Study the drawing (mm; zero at the part's minimum x, y, z) and answer. A direction names the side the tool comes from. Give positions to 0.01 mm unless a question says otherwise; leave off trailing zeros. Order: outer loops, then holes, each group sorted by start corner. A loop starts at its lowest first (then second) coordinate and runs counter-clockwise, first axis right, second up. Notation, with made-up numbers: (67.25, 3.25) - (119.25, 3.25) arc R37 ccw to (119.25, 40.25) - close; hole circle Ø7 at (77.25, -23.75). An arc over 180 degrees is marked (long way). Write each question's results on one line, items separated by ' | '. Start each with the question number.
1. Section D-D (z = 1.25) is taken. Give the vertices of the cut face in (x, y), and give its area (3 significant figures).
2. Find the intervals of material crossed by L1, parallel to X at y = 9.75, z = 2.25; L2, parallel to Z at x = 3.75, y = 16.75; L3, parallel to Z at x = 9, y = 9.25, in increasing order.
3. Determine the mould class of the marked faces 3, 4 and 5 for opening direction X: released by +X, released by -X, zero draft, split by the parting line, or undercut.
4. Which of the six approach directions +Z, -Z, +X, -X, +Y, -Y give full straight-line access (tool end or side, diameter ignored) to the marked faces 1 and 2?
5. Section B-B (x = 7.5) is taken. Give the vertices of the cut face in (y, z), and give its area (3 significant figures).
6. Flat-ended cylindrical pins translate along their axes: pin 1 (5 mm diameter, centred on x = 15.5, y = 17, fed in from +Z); pin 2 (1 mm diameter, centred on x = 12, z = 1, fed in from +Y); pin 3 (1.5 mm diameter, centred on x = 10.5, y = 10, fed in from +Z). Find the tip coordinate at first contact, or state that the pin passes through.
7. Section C-C (z = 2.25) is taken. Give the vertices of the cut face in (x, y), and give its area (3 significant figures).
8. Section A-A (y = 8) is taken. Give the vertices of the cut face in (x, z).
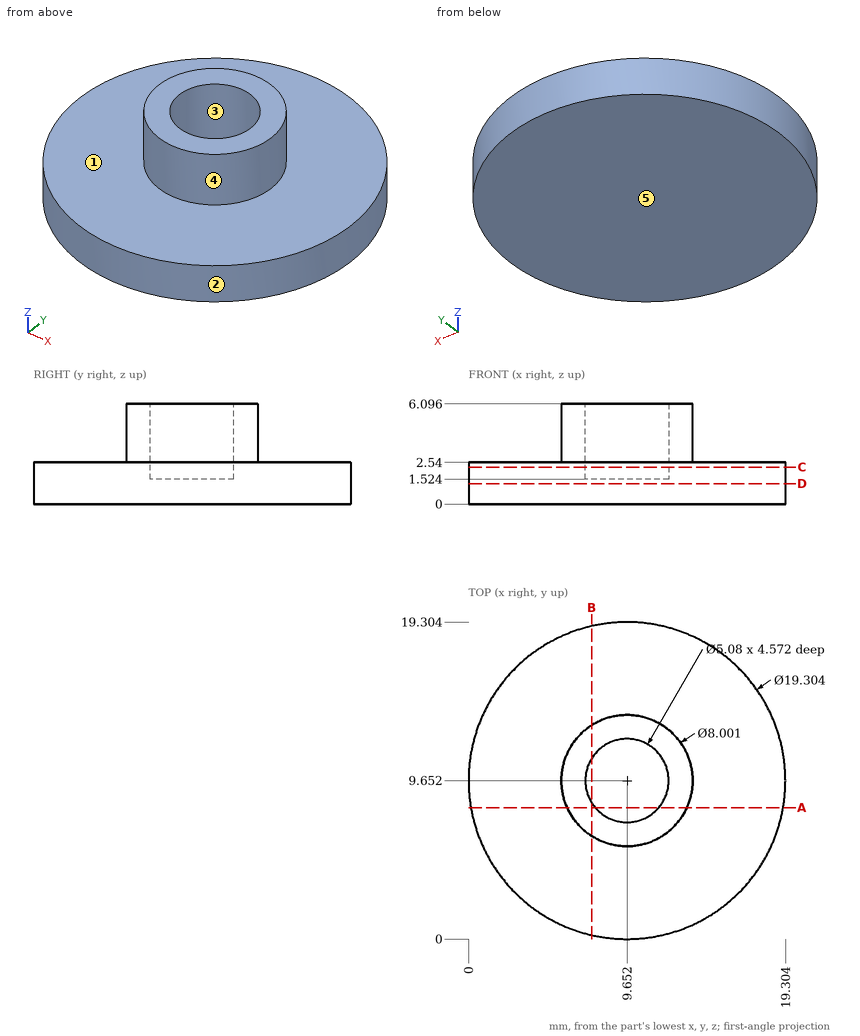
Reported:
1) outline: circle Ø19.3 at (9.65, 9.65) | area: 293 mm²
2) L1: 0 to 7.11, 12.19 to 19.3 | L2: 0 to 2.54 | L3: 0 to 1.52
3) face 3: undercut | face 4: split by the parting line | face 5: zero draft
4) face 1: +Z | face 2: +Z, -Z
5) outline: (0.24, 0) - (19.06, 0) - (19.06, 2.54) - (13.02, 2.54) - (13.02, 6.1) - (11, 6.1) - (11, 1.52) - (8.3, 1.52) - (8.3, 6.1) - (6.28, 6.1) - (6.28, 2.54) - (0.24, 2.54) - close | area: 59.4 mm²
6) pin 1: z = 2.54 | pin 2: y = 19.13 | pin 3: z = 1.52
7) outline: circle Ø19.3 at (9.65, 9.65); hole circle Ø5.08 at (9.65, 9.65) | area: 272 mm²
8) outline: (0.14, 0) - (19.16, 0) - (19.16, 2.54) - (13.3, 2.54) - (13.3, 6.1) - (11.58, 6.1) - (11.58, 1.52) - (7.72, 1.52) - (7.72, 6.1) - (6.01, 6.1) - (6.01, 2.54) - (0.14, 2.54) - close
